Could you check a few things on this model? Use its own coordinates, in mm. Face numbers are marked on the shaded views. Round coordinates to 2 decimals unless told otherwise and drop trailing zeros. Loops run counter-clockwise (first coordinate to the right, second up) from the corner with the lowest first, then second, coordinate; pieces in that order, holes last. Notation, with made-up numbers: (64.25, -14.5) -> (77.25, -14.5) arc R34 cw to (77.25, 18.5) -> close; hole circle Ø11 at (20, -5). An arc over 180 degrees is marked (long way). One line per item, written item: value.
```python
from build123d import *

# Parameters (mm, degrees)
SKETCH2_R          = 3
CUT_EXTRUDE1_DEPTH = 23
SKETCH3_R          = 3.25
SKETCH3_R_2        = 3.4
SKETCH3_R_3        = 3.697443322
CUT_EXTRUDE2_DEPTH = 23


with BuildPart() as part:
    # Sketch1 → Revolve1 (revolve)
    with BuildSketch(Plane(origin=(0, 0, 0), x_dir=(0, 0, -1), z_dir=(1, 0, 0)), mode=Mode.PRIVATE) as revolve1_sk:
        Polygon((0.25, 15.75), (5, 15.75), (5, 29.75), (5.25, 30), (72.75, 30), (73, 29.75), (73, 28.85), (72, 28.85), (72, 26.85), (73, 26.85), (73, 14.85), (72.75, 14.6), (12.575, 14.6), (12, 14.025), (6.5, 14.025), (6.5, 8.75), (6.25, 8.5), (3.55, 8.5), (3.3, 8.75), (3.3, 11.525), (0.25, 11.525), (0, 11.775), (0, 15.5), align=None)
    revolve(revolve1_sk.sketch.rotate(Axis((0, 0, 0), (0, 0, -1)), 90), axis=Axis((0, 0, 0), (0, 0, -1)))

    # Sketch2 → Cut-Extrude1 (cut)
    with BuildSketch(Plane.XY.offset(-5)):
        with Locations((15.909902577, -15.909902577)):
            Circle(SKETCH2_R)
        with Locations((-15.909902577, -15.909902577)):
            Circle(SKETCH2_R)
        with Locations((0, 22.5)):
            Circle(SKETCH2_R)
    extrude(amount=-CUT_EXTRUDE1_DEPTH, mode=Mode.SUBTRACT)

    # Sketch3 → Cut-Extrude2 (cut)
    with BuildSketch(Plane(origin=(0, 0, -73), x_dir=(-1, 0, 0), z_dir=(0, 0, -1))):
        with Locations((0, -19.763693495)):
            Circle(SKETCH3_R)
        with Locations((-18.796389484, -6.107317162)):
            Circle(SKETCH3_R)
        with Locations((-11.616807567, 15.989163909)):
            Circle(SKETCH3_R)
        with Locations((11.616807567, 15.989163909)):
            Circle(SKETCH3_R)
        with Locations((18.796389484, -6.107317162)):
            Circle(SKETCH3_R)
        with Locations((0, 21.2)):
            Circle(SKETCH3_R_2)
        with Locations((-12.45, -17.15)):
            Circle(SKETCH3_R_2)
        with Locations((12.45, -17.15)):
            Circle(SKETCH3_R_2)
        with Locations((-20.112696309, 6.901022254)):
            Circle(SKETCH3_R_3)
        with Locations((20.112696309, 6.901022254)):
            Circle(SKETCH3_R_3)
    extrude(amount=-CUT_EXTRUDE2_DEPTH, mode=Mode.SUBTRACT)


solid = part.part
```
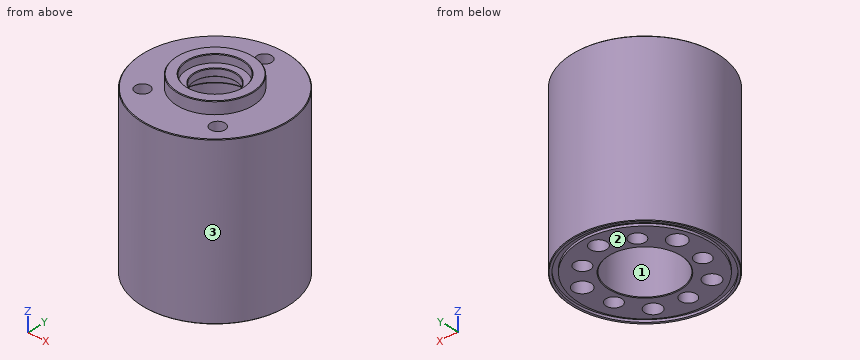
(1) For pin 1 Ø5.5 at (x, y) = (-12.5, -15.5) entering from -Z; pin 2 Ø2 at (y, z) = (16, -9.5) entering from -X; pin 3 Ø3 at (x, y) = (-15, -15) entering from +Z; pin 4 Ø3 at (y, z) = (15.5, -50) entering from +X, each with a flat end and sliding along its axis, tell me the tip position at first contact or that it passes through.
Results below:
pin 1: stops at z = -73
pin 2: stops at x = -25.98
pin 3: stops at z = -28
pin 4: stops at x = 26.53
(2) Please list where these lines run through material, in increasing order: L1, parallel to Y at x = 0, z = -9.5 (3 decimals); L2, parallel to X at y = -17, z = -55; L3, parallel to Y at x = 13, z = -64.
Results below:
L1: y = -30 to -14.025, 14.025 to 19.5, 25.5 to 30
L2: x = -24.72 to -15.85, -9.05 to -1.71, 1.71 to 9.05, 15.85 to 24.72
L3: y = -27.04 to -20.51, -13.79 to -6.65, 6.65 to 13.05, 18.93 to 27.04
(3) Imagine slicing it at B-B on z = -31. Write out the boundary of the cut face in (x, y), then the cut area to 3 significant figures.
Results below:
outline: circle Ø60 at (0, 0); hole circle Ø29.2 at (0, 0)
area: 2,160 mm²
(4) We'd pull the mould along Y, two halves only. Please class the marked faces 1, 2 and 3: +Y half, -Y half, draft (parallel to the pull), parting line (faces both ways), or undercut.
Results below:
face 1: undercut
face 2: draft
face 3: parting line
(5) Imagine slicing it at A-A on z = -64.5. Give the number of separate pieces and of enclosed holes in the cut face, then the cut area to 3 significant figures.
Results below:
separate pieces: 1
enclosed holes: 11
area: 1,800 mm²
(6) Imagine slicing it at C-C on z = -15. Write out the boundary of the cut face in (x, y).
Results below:
outline: circle Ø60 at (0, 0); hole circle Ø6 at (-15.91, -15.91); hole circle Ø29.2 at (0, 0); hole circle Ø6 at (0, 22.5); hole circle Ø6 at (15.91, -15.91)
